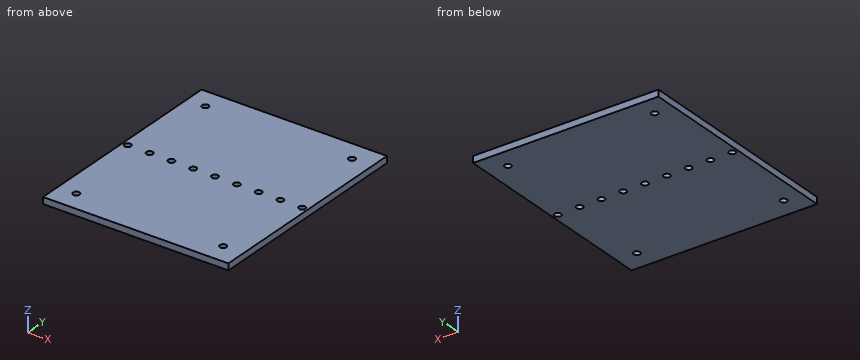
```python
from build123d import *

# Parameters (mm, degrees)
SKETCH1_W           = 85
SKETCH1_H           = 100
BOSS_EXTRUDE1_DEPTH = 3
SKETCH2_R           = 1.5
CUT_EXTRUDE1_DEPTH  = 4
SKETCH3_R           = 1.5
CUT_EXTRUDE2_DEPTH  = 10


with BuildPart() as part:
    # Sketch1 → Boss-Extrude1 (new body)
    with BuildSketch(Plane.XY):
        with Locations((42.5, 0)):
            Rectangle(SKETCH1_W, SKETCH1_H)
    extrude(amount=BOSS_EXTRUDE1_DEPTH)

    # Sketch2 → Cut-Extrude1 (cut)
    with BuildSketch(Plane.XY.offset(3)):
        with Locations((75.8, 40.64)):
            Circle(SKETCH2_R)
        with Locations((75.8, -40.64)):
            Circle(SKETCH2_R)
        with Locations((8.49, 40.64)):
            Circle(SKETCH2_R)
        with Locations((8.49, -40.64)):
            Circle(SKETCH2_R)
    extrude(amount=-CUT_EXTRUDE1_DEPTH, mode=Mode.SUBTRACT)

    # Sketch3 → Cut-Extrude2 (cut)
    with BuildSketch(Plane.XY.offset(3)):
        with Locations((42.5, 0)):
            Circle(SKETCH3_R)
        with Locations((52.5, 0)):
            Circle(SKETCH3_R)
        with Locations((62.5, 0)):
            Circle(SKETCH3_R)
        with Locations((72.5, 0)):
            Circle(SKETCH3_R)
        with Locations((82.5, 0)):
            Circle(SKETCH3_R)
        with Locations((32.5, 0)):
            Circle(SKETCH3_R)
        with Locations((22.5, 0)):
            Circle(SKETCH3_R)
        with Locations((12.5, 0)):
            Circle(SKETCH3_R)
        with Locations((2.5, 0)):
            Circle(SKETCH3_R)
    extrude(amount=-CUT_EXTRUDE2_DEPTH, mode=Mode.SUBTRACT)


solid = part.part
```
Here's how the part is built. I have some questions about the finished solid (model axes, mm). Coordinates: 2 decimals unless noted, no trailing zeros. Order: outer loops, then holes, each group sorted by start corner. A loop starts at its lowest first (then second) coordinate and runs counter-clockwise, first axis right, second up.
Item 1: I'm going to push a flat-ended pin straight in: pin 1 Ø2.5 at (x, y) = (82.5, 0) entering from +Z. Where does the tip first touch, or does it pass through?
Response values:
pin 1: passes through
Item 2: I need wall thicknesses on probe 1 along Y at (x, z) = (75.8, 2.35); probe 2 along Y at (x, z) = (22.5, 1.45); probe 3 along Y at (x, z) = (9, 2.5). Which ranges of each line are inside material? Lowest first, please.
Response values:
probe 1: y = -50 to -42.14, -39.14 to 39.14, 42.14 to 50
probe 2: y = -50 to -1.5, 1.5 to 50
probe 3: y = -50 to -42.05, -39.23 to 39.23, 42.05 to 50
Item 3: If we section it at B-B, the plane x = 82.5: List the corners of the cut face in (y, z) for me.
Response values:
outline: (-50, 0) - (-1.5, 0) - (-1.5, 3) - (-50, 3) - close; (1.5, 0) - (50, 0) - (50, 3) - (1.5, 3) - close
Item 4: If we section it at A-A, the plane y = -40.64: List the corners of the cut face in (x, z) for me.
Response values:
outline: (0, 0) - (6.99, 0) - (6.99, 3) - (0, 3) - close; (9.99, 0) - (74.3, 0) - (74.3, 3) - (9.99, 3) - close; (77.3, 0) - (85, 0) - (85, 3) - (77.3, 3) - close
